Verification items for the finished model (mm, model axes). A direction names the side the tool comes from. Round coordinates to 2 decimals unless told otherwise and drop trailing zeros. Write each loop counter-clockwise with the first axis right and the second up, starting at its lowest first coordinate (ties: lowest second). Pieces come first, ordered by that corner, then holes. Notation, with made-up numbers: (21.5, 18.5) -> (49.5, 18.5) arc R27 ccw to (49.5, 34.5) -> close; hole circle Ø5 at (-15.75, 73). An arc over 180 degrees is marked (long way). Use CSV: the item, a comma, the result in double quotes.
Autodesk Inventor part; units mm, degrees
ref_plane "YZ Plane" through (0, 0, 0) normal (1, 0, 0) x (0, 1, 0)
ref_plane "XZ Plane" through (0, 0, 0) normal (0, 1, 0) x (-1, 0, 0)
ref_plane "XY Plane" through (0, 0, 0) normal (0, 0, 1) x (1, 0, 0)
sketch "Sketch1" plane through (0, 0, 0) normal (0, 0, 1) x (1, 0, 0)
  circle A0 centre (0, 0) radius 2.00025
  dimension "d0" = 4.0005
extrude "Extrusion1" add sketch "Sketch1" along normal blind 75
sketch "Sketch2" plane through (0, 0, 0) normal (0, 0, 1) x (1, 0, 0)
  circle A0 centre (0, 0) radius 2.00025
  line L0 (1.353027, 1.4732) -> (-1.353027, 1.4732)
  line L1 (0, 2.80035) -> (0, -2.80035)
  line L2 (-2.80035, 0) -> (2.80035, 0)
  line L3 (1.723004, 1.016) -> (-1.723004, 1.016)
  line L4 (0.7112, 1.016) -> (1.18047, 0.2032)
  line L5 (1.18047, 0.2032) -> (-1.18047, 0.2032)
  line L6 (-1.18047, 0.2032) -> (-0.7112, 1.016)
  line L7 (0, 0) -> (0, 2.00025)
  dimension "d6" = 1.016
  dimension "d9" = 60
  dimension "d10" = 1.4224
  dimension "d11" = 0.8128
  dimension "d40" = 0.4572
extrude "Extrusion3" cut sketch "Sketch2" along normal blind 9.525 contours L3 L1 L0 A0 | L1 L3 A0 L0
extrude "Extrusion4" cut sketch "Sketch2" along normal blind 8.763 contours L4 L5 L1 L3 | L5 L6 L3 L1
sketch "Sketch3" plane through (-1.18047, 0.2032, 9.525) normal (0, 1, 0) x (1, 0, 0)
  line L0 (0, 9.525) -> (2.360941, 9.525)
  line L1 (1.18047, 24.525) -> (1.18047, -80.475)
  point P0 (1.18047, 9.525)
  point P1 (1.18047, 5.334)
  dimension "d14" = 4.191
hole "Hole1" at (0, 0.2032, 4.191) direction (0, -1, 0) diameter 1.2192 end through all
sketch "Sketch4" plane through (0, 0, 0) normal (1, 0, 0) x (0, 1, 0)
  line L0 (0, 120) -> (0, -20)
  line L1 (-2.00025, 0) -> (-2.00025, 75)
  line L2 (0, 0) -> (-2.00025, 3.464535)
  line L3 (-2.00025, 3.464535) -> (-2.00025, 0)
  line L4 (-2.00025, 0) -> (0, 0)
  dimension "d23" = 30
extrude "Extrusion5" cut sketch "Sketch4" along normal mid plane 12.7
chamfer "Chamfer1" distance 0.254 distance2 0.381 1 edges at (-0.9458, 0.6096, 0) measured on face at (-1.2049, 0.7451, 0)
chamfer "Chamfer2" distance 0.254 distance2 0.381 1 edges at (0.9458, 0.6096, 0) measured on face at (1.2049, 0.7451, 0)
chamfer "Chamfer3" distance 0.381 angle 45 1 edges at (-2.0003, 0, 75)
extrude "Extrusion7" cut sketch "Sketch2" along normal blind 25.4 contours L3 L1 L0 A0 | L0 L1 A0 | L1 L0 A0 | L1 L3 A0 L0
sketch "Sketch6" plane through (-0.7112, 1.016, 9.525) normal (0, 1, 0) x (1, 0, 0)
  line L0 (-1.011804, -15.875) -> (2.434204, -15.875)
  line L1 (0.7112, 24.525) -> (0.7112, -80.475)
  line L2 (6.9342, 9.525) -> (-5.5118, 9.525)
  line L3 (5.1562, -1.143) -> (-3.7338, -1.143)
  line L4 (-3.7338, -1.143) -> (-3.7338, -15.875)
  line L5 (-3.7338, -15.875) -> (5.1562, -15.875)
  line L6 (5.1562, -15.875) -> (5.1562, -1.143)
  line L7 (5.1562, -1.143) -> (-3.7338, -15.875) construction
  line L8 (-3.7338, -1.143) -> (5.1562, -15.875) construction
  point P0 (0.7112, 9.525)
  point P1 (0.7112, -8.509)
  dimension "d43" = 0
  dimension "d45" = 8.89
  dimension "d68" = 10.668
  dimension "d69" = 14.732
extrude "Extrusion8" cut sketch "Sketch6" against normal blind 0.508
sketch "Sketch11" plane through (0, 0, 0) normal (1, 0, 0) x (0, 1, 0)
  line L0 (0.508, 10.668) -> (0.508, 25.4)
  line L1 (2.00025, 25.4) -> (2.00025, 74.619)
  line L2 (0.635, 25.4) -> (2.00025, 27.764682)
  line L3 (0.508, 10.668) -> (1.016, 10.668)
  line L4 (-0.40005, 0) -> (2.4003, 0)
  line L5 (0.635, 10.668) -> (1.016, 10.008089)
  line L6 (1.016, 10.008089) -> (1.016, 10.668)
  line L7 (0.635, 10.668) -> (1.016, 10.668)
  line L8 (2.00025, 27.764682) -> (2.00025, 25.4)
  line L9 (2.00025, 25.4) -> (0.508, 25.4)
  line L10 (0.635, 25.4) -> (2.00025, 25.4)
  point P0 (0, 0)
  dimension "d56" = 0.127
  dimension "d57" = 10.668
  dimension "d58" = 0.127
  dimension "d59" = 30
  dimension "d64" = 30
extrude "Extrusion10" cut sketch "Sketch11" along normal mid plane 6.35
sketch "Sketch12" plane through (-1.473764, 0.2032, 0) normal (0, 1, 0) x (1, 0, 0)
  circle A0 centre (1.473764, -4.191) radius 0.6096
  circle A1 centre (1.473764, -4.191) radius 0.8
  circle A2 centre (1.473764, -4.191) radius 0.7
  point P0 (1.473764, 0)
  dimension "d65" = 1.6
  dimension "d66" = 1.4
sketch "Sketch14" plane through (0, 0, 8.763) normal (0, 0, -1) x (-1, 0, 0)
  line L0 (0.7112, 1.016) -> (1.18047, 0.2032)
  line L1 (-1.473764, 0.2032) -> (1.473764, 0.2032)
  line L2 (0.7112, 1.016) -> (0.7112, 0.2032)
  line L3 (1.18047, 0.2032) -> (-1.18047, 0.2032)
  line L4 (0.7112, 0.2032) -> (1.18047, 0.2032)
  line L5 (0, -2.80035) -> (0, 2.80035)
  line L6 (0, 0.2032) -> (0, 1.016)
  line L7 (0.7112, 1.016) -> (0, 1.016)
  line L8 (0, 1.016) -> (0, 0.2032)
  line L9 (0, 0.2032) -> (0.7112, 0.2032)
  line L10 (0.7112, 0.2032) -> (0.7112, 1.016)
  point P0 (0, 0)
revolve "Revolution1" cut sketch "Sketch14" angle 360 about axis through (0, 0, 8.763) along (0, 1, 0)
properties part number "J008040 NEUROPIXELS GEN 2 DOVE TAIL PROBE HOLDER Rev -" material "ALUMINUM, 7075-T651"
Q1. Material ranges on L1, parallel to X at y = 0.65, z = 40.5; L2, parallel to Y at x = 0.6, z = 56; L3, parallel to Z at x = 0, y = -0.4, recorded low to high.
Filled in:
L1,"-1.89 to 1.89"
L2,"-1.91 to 1.91"
L3,"0.69 to 3.58, 4.8 to 75"
Q2. Go/stop test with flat-tipped pins: P1, Ø1.6, axis at x = 0, z = 4.191, coming from the +Y side; P2, Ø1.2, axis at x = 0.5, z = 15, coming from the +Y side. Record where each tip stops, or that it passes through.
Filled in:
P1,"y = 1.02"
P2,"y = 0.51"
Q3. Section check B-B (z = 30.5). Record the cut outline in (x, y).
Filled in:
outline,"circle Ø4 at (0, 0)"
Q4. Section check A-A (x = 0). Record the cut outline in (y, z) (3 decimals).
Filled in:
outline,"(-2, 3.465) -> (0, 0) -> (0.203, 0) -> (0.203, 3.581) -> (-2, 3.581) -> close; (-2, 4.801) -> (0.203, 4.801) -> (0.203, 9.943) -> (1.016, 9.474) -> (1.016, 10.008) -> (0.635, 10.668) -> (0.508, 10.668) -> (0.508, 25.4) -> (0.635, 25.4) -> (2, 27.765) -> (2, 74.619) -> (1.619, 75) -> (-1.619, 75) -> (-2, 74.619) -> close"
Q5. Mould release check, pull along X, two halves, no side actions. Record for faces 1 (the flat face through (-0.027, 1.156, 26.303)), 2 (the cylindrical face through (0, -2, 37)), 3 (the flat face through (0, 0.203, 5)), 4 (the conical face through (0, 0.8, 9.6)): released by +X, released by -X, zero draft, split by the parting line, or undercut.
Filled in:
face 1,"zero draft"
face 2,"split by the parting line"
face 3,"undercut"
face 4,"undercut"
Q6. Access from +Z, -Z, +X, -X, +Y, -Y to the whole of each face (thin tool, end or side, straight path). Record for faces 5 (the cylindrical face through (0.371, -0.914, 3.707)), 6 (the flat face through (1, 1.016, 5)), 7 (the flat face through (0, 0.508, 18)).
Filled in:
face 5,"+Y, -Y"
face 6,"-Z, +X, -X, +Y"
face 7,"+X, -X, +Y"
